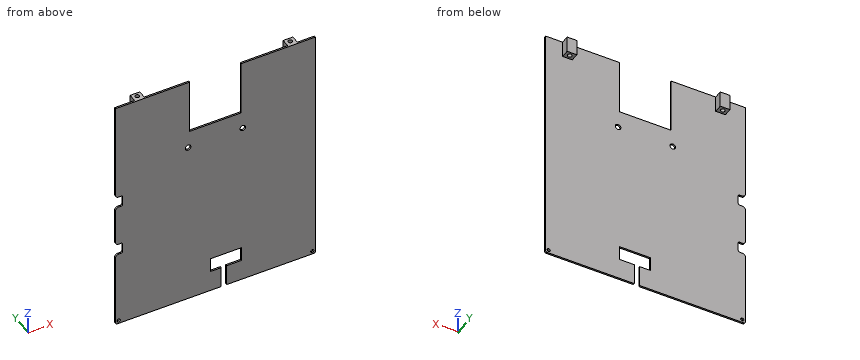
Autodesk Inventor part; units mm, degrees
ref_plane "YZ Plane" through (0, 0, 0) normal (1, 0, 0) x (0, 1, 0)
ref_plane "XZ Plane" through (0, 0, 0) normal (0, 1, 0) x (-1, 0, 0)
ref_plane "XY Plane" through (0, 0, 0) normal (0, 0, 1) x (1, 0, 0)
sketch "Sketch1" plane through (0, 0, 0) normal (0, 1, 0) x (-1, 0, 0)
  line L0 (-90.1493, 193.0734) -> (34.8507, 193.0734) construction
  line L1 (34.8507, 193.0734) -> (34.8507, 51.5734) construction
  line L2 (34.8507, 51.5734) -> (28.8507, 51.5734) construction
  line L3 (28.8507, 51.5734) -> (28.8507, 31.5734) construction
  line L4 (34.8507, 31.5734) -> (28.8507, 31.5734) construction
  line L5 (34.8507, 31.5734) -> (34.8507, -109.9266) construction
  line L6 (34.8507, -109.9266) -> (-90.1493, -109.9266) construction
  line L7 (-90.1493, -109.9266) -> (-90.1493, 31.5734) construction
  line L8 (-90.1493, 31.5734) -> (-84.1493, 31.5734) construction
  line L9 (-84.1493, 51.5734) -> (-84.1493, 31.5734) construction
  line L10 (-90.1493, 51.5734) -> (-84.1493, 51.5734) construction
  line L11 (-90.1493, 51.5734) -> (-90.1493, 193.0734) construction
  line L12 (-91.6493, 194.5734) -> (-91.6493, -111.4266) construction
  line L13 (-91.6493, -111.4266) -> (36.3507, -111.4266) construction
  line L14 (36.3507, -111.4266) -> (36.3507, 194.5734) construction
  line L15 (36.3507, 194.5734) -> (-91.6493, 194.5734) construction
  circle A0 centre (-88.1493, -107.9266) radius 1.1 construction
  line L16 (-86.1493, -109.9266) -> (-90.1493, -109.9266) construction
  line L17 (-86.1493, -109.9266) -> (-86.1493, -105.9266) construction
  line L18 (-86.1493, -105.9266) -> (-90.1493, -105.9266) construction
  line L19 (-90.1493, -109.9266) -> (-90.1493, -105.9266) construction
  line L20 (34.8507, -109.9266) -> (30.8507, -109.9266) construction
  line L21 (34.8507, -105.9687) -> (34.8507, -109.9266) construction
  line L22 (34.8507, -105.9687) -> (30.8507, -105.9687) construction
  line L23 (30.8507, -105.9687) -> (30.8507, -109.9266) construction
  circle A1 centre (32.8507, -107.9687) radius 1.1 construction
  circle A2 centre (-88.1493, 191.0734) radius 1.1 construction
  line L24 (-90.1493, 189.0734) -> (-90.1493, 193.0734) construction
  line L25 (-90.1493, 189.0734) -> (-86.1493, 189.0734) construction
  line L26 (-86.1493, 189.0734) -> (-86.1493, 193.0734) construction
  line L27 (-90.1493, 193.0734) -> (-86.1493, 193.0734) construction
  circle A3 centre (32.8507, 191.0734) radius 1.1 construction
  line L28 (30.8507, 193.0734) -> (34.8507, 193.0734) construction
  line L29 (30.8507, 193.0734) -> (30.8507, 189.0734) construction
  line L30 (30.8507, 189.0734) -> (34.8507, 189.0734) construction
  line L31 (34.8507, 193.0734) -> (34.8507, 189.0734) construction
  point P0 (0, 0)
  point P1 (0, 0)
sketch "Sketch2" plane through (0, 0, 0) normal (0, 1, 0) x (-1, 0, 0)
  line L0 (-89.7618, 28.8226) -> (-89.7618, 191.8096)
  line L1 (-88.7618, 192.8096) -> (33.3754, 192.8096)
  line L2 (34.3754, 191.8096) -> (34.3754, -108.6932)
  line L3 (-89.7618, -108.6932) -> (-89.7618, 28.8226)
  circle A0 centre (-87.7618, -107.6932) radius 1
  circle A1 centre (32.3754, -107.6932) radius 1
  line L4 (34.3754, 28.9308) -> (34.3754, -108.6932)
  circle A2 centre (-87.7618, 190.8096) radius 1
  circle A3 centre (32.3754, 190.8096) radius 1
  arc A4 (34.3754, 191.8096) -> (33.3754, 192.8096) centre (33.3754, 191.8096) ccw
  arc A5 (-88.7618, 192.8096) -> (-89.7618, 191.8096) centre (-88.7618, 191.8096) ccw
  arc A6 (-89.7618, -108.6932) -> (-88.7618, -109.6932) centre (-88.7618, -108.6932) ccw
  arc A7 (33.3754, -109.6932) -> (34.3754, -108.6932) centre (33.3754, -108.6932) ccw
  line L5 (-43.6932, 76.0582) -> (-11.6932, 76.0582)
  line L6 (-11.6932, 76.0582) -> (-11.6932, 7.0582)
  line L7 (-11.6932, 7.0582) -> (-43.6932, 7.0582)
  line L8 (-43.6932, 7.0582) -> (-43.6932, 76.0582)
  circle A8 centre (-44.6932, 80.8582) radius 1.75
  circle A9 centre (-10.6932, 80.8582) radius 1.75
  circle A10 centre (-10.6932, -3.9418) radius 1.75
  circle A11 centre (-44.6932, -3.9418) radius 1.75
  line L9 (-43.8518, -87.5066) -> (-24.58, -87.5066)
  line L10 (-24.58, -87.5066) -> (-24.58, -96.4362)
  line L11 (-43.8518, -96.4362) -> (-43.8518, -87.5066)
  line L12 (-34.6195, -96.4362) -> (-34.6195, -109.6932)
  line L13 (-31.2888, -109.6932) -> (-31.2888, -96.4362)
  line L14 (-24.58, -96.4362) -> (-31.2888, -96.4362)
  line L15 (-34.6195, -96.4362) -> (-43.8518, -96.4362)
  line L16 (33.3754, -109.6932) -> (-31.2888, -109.6932)
  line L17 (-34.6195, -109.6932) -> (-88.7618, -109.6932)
  line L18 (34.0825, -109.4003) -> (-89.4689, 192.5167) construction
  line L19 (-89.4689, -109.4003) -> (34.0825, 192.5167) construction
  line L20 (-27.6932, 41.5582) -> (9.3943, 41.5582) construction
  point P0 (0, 0)
  point P1 (-89.7618, 188.8096)
  point P2 (-85.7618, 192.8096)
  point P3 (-89.7618, 192.8096)
  dimension "d3" = 1
  dimension "d47" = 69
  dimension "d48" = 32
  dimension "d52" = 34.5
  dimension "d53" = 16
  dimension "d54" = 3.5
  dimension "d55" = 3.5
  dimension "d56" = 3.5
  dimension "d57" = 3.5
  dimension "d59" = 0
  dimension "d62" = 0
  dimension "d64" = 0
  dimension "d65" = 0
  dimension "d66" = 11
  dimension "d67" = 4.8
  dimension "d68" = 1
  dimension "d69" = 1
  dimension "d87" = 2
  dimension "d88" = 2
  dimension "d89" = 2
  dimension "d90" = 2
  dimension "d91" = 2
  dimension "d92" = 2
  dimension "d93" = 2
  dimension "d94" = 2
  dimension "d95" = 2
  dimension "d96" = 2
  dimension "d97" = 2
  dimension "d98" = 2
extrude "Extrusion1" add sketch "Sketch2" along normal blind 1
ref_plane "Work Plane1" through (-33.3754, 0, 41.5582) normal (0, 0, 1) x (1, 0, 0)
sketch "Sketch4" plane through (0, 1, 0) normal (0, 1, 0) x (1, 0, 0)
  line L0 (79.1186, -31.5582) -> (73.1186, -31.5582)
  line L1 (73.1186, -31.5582) -> (73.1186, -51.5582)
  line L2 (73.1186, -51.5582) -> (79.1186, -51.5582)
  line L3 (79.1186, -51.5582) -> (79.1186, -31.5582)
  line L4 (117.2493, -41.5582) -> (-61.9507, -41.5582)
  line L5 (-15.9231, -31.5582) -> (-21.9231, -31.5582)
  line L6 (-21.9231, -31.5582) -> (-21.9231, -51.5582)
  line L7 (-21.9231, -51.5582) -> (-15.9231, -51.5582)
  line L8 (-15.9231, -51.5582) -> (-15.9231, -31.5582)
  dimension "d10" = 6
  dimension "d11" = 20
  dimension "d12" = 10
  dimension "d13" = 6
  dimension "d14" = 20
  dimension "d15" = 10
extrude "Extrusion2" add sketch "Sketch4" along normal blind 5
sketch "Sketch6" plane through (-21.9231, 1, 51.5582) normal (0, 0, 1) x (1, 0, 0)
  line L0 (0, 5) -> (6, 5)
  line L1 (0, 0) -> (0, 5)
  line L2 (95.0417, 5) -> (101.0417, 5)
  line L3 (95.0417, 0) -> (95.0417, 5)
  point P0 (21.9231, -1)
  point P1 (3, 2.5)
  point P2 (98.0417, 2.5)
  dimension "d22" = 2.5
  dimension "d23" = 3
  dimension "d24" = 2.5
  dimension "d25" = 3
hole "Hole1" at (-18.9231, 3.5, 51.5582) at (76.1186, 3.5, 51.5582) direction (0, 0, -1) diameter 2.6 depth 5 countersink diameter 5 countersink angle 82
sketch "Sketch7" plane through (-18.9231, 3.5, 46.5582) normal (0, 0, 1) x (1, 0, 0)
  circle A0 centre (0, 0) radius 1.3
  point P0 (18.9231, -3.5)
hole "Hole2" at (-18.9231, 3.5, 46.5582) direction (0, 0, -1) diameter 2.6 depth 15 tip angle 118
sketch "Sketch8" plane through (76.1186, 3.5, 46.5582) normal (0, 0, 1) x (1, 0, 0)
  circle A0 centre (0, 0) radius 1.3
  point P0 (-76.1186, -3.5)
hole "Hole3" at (76.1186, 3.5, 46.5582) direction (0, 0, -1) diameter 2.6 depth 15 tip angle 118
sketch "Sketch9" plane through (0, 0, 0) normal (0, -1, 0) x (1, 0, 0)
  line L0 (-34.3754, -108.6932) -> (-34.3754, 191.8096)
  line L1 (-34.3754, 137.8096) -> (-30.8754, 137.8096)
  line L2 (-29.8754, 136.8096) -> (-29.8754, 131.8096)
  line L3 (-30.8754, 130.8096) -> (-34.3754, 130.8096)
  line L4 (-34.3754, 130.8096) -> (-34.3754, 137.8096)
  line L5 (-34.3754, 104.8096) -> (-30.8754, 104.8096)
  line L6 (-29.8754, 103.8096) -> (-29.8754, 98.8096)
  line L7 (-30.8754, 97.8096) -> (-34.3754, 97.8096)
  line L8 (-34.3754, 97.8096) -> (-34.3754, 104.8096)
  line L9 (-34.3754, -21.1904) -> (-30.8754, -21.1904)
  line L10 (-29.8754, -22.1904) -> (-29.8754, -27.1904)
  line L11 (-30.8754, -28.1904) -> (-34.3754, -28.1904)
  line L12 (-34.3754, -28.1904) -> (-34.3754, -21.1904)
  line L13 (-34.3754, -54.1904) -> (-30.8754, -54.1904)
  line L14 (-29.8754, -55.1904) -> (-29.8754, -60.1904)
  line L15 (-30.8754, -61.1904) -> (-34.3754, -61.1904)
  line L16 (-34.3754, -61.1904) -> (-34.3754, -54.1904)
  line L17 (-33.3754, 192.8096) -> (88.7618, 192.8096)
  arc A0 (-29.8754, 136.8096) -> (-30.8754, 137.8096) centre (-30.8754, 136.8096) ccw
  arc A1 (-30.8754, 130.8096) -> (-29.8754, 131.8096) centre (-30.8754, 131.8096) ccw
  arc A2 (-29.8754, 103.8096) -> (-30.8754, 104.8096) centre (-30.8754, 103.8096) ccw
  arc A3 (-30.8754, 97.8096) -> (-29.8754, 98.8096) centre (-30.8754, 98.8096) ccw
  arc A4 (-29.8754, -22.1904) -> (-30.8754, -21.1904) centre (-30.8754, -22.1904) ccw
  arc A5 (-30.8754, -28.1904) -> (-29.8754, -27.1904) centre (-30.8754, -27.1904) ccw
  arc A6 (-29.8754, -55.1904) -> (-30.8754, -54.1904) centre (-30.8754, -55.1904) ccw
  arc A7 (-30.8754, -61.1904) -> (-29.8754, -60.1904) centre (-30.8754, -60.1904) ccw
  point P0 (0, 0)
  point P1 (-29.8754, 97.8096)
  point P2 (-29.8754, 104.8096)
  point P3 (-29.8754, -28.1904)
  point P4 (-29.8754, -21.1904)
  point P5 (-29.8754, -61.1904)
  point P6 (-29.8754, -54.1904)
  dimension "d70" = 55
  dimension "d71" = 7
  dimension "d72" = 7
  dimension "d73" = 26
  dimension "d74" = 26
  dimension "d75" = 7
  dimension "d76" = 7
  dimension "d77" = 119
  dimension "d78" = 4.5
  dimension "d79" = 4.5
  dimension "d80" = 1
  dimension "d81" = 1
extrude "Extrusion3" cut sketch "Sketch9" against normal through all
fillet "Fillet1" radius 2 8 edges at (-34.3754, 0.5, 137.8096) (-34.3754, 0.5, 130.8096) (-34.3754, 0.5, 104.8096) (-34.3754, 0.5, 97.8096) (-34.3754, 0.5, -21.1904) (-34.3754, 0.5, -28.1904) (-34.3754, 0.5, -54.1904) (-34.3754, 0.5, -61.1904)
sketch "Sketch11" plane through (0, 0, 0) normal (0, -1, 0) x (1, 0, 0)
  line L0 (-34.3754, 139.8096) -> (-34.3754, 191.8096)
  line L1 (-34.3754, 178.177) -> (-25.2482, 178.177)
  line L2 (-25.2482, 178.177) -> (-25.2482, 158.3724)
  line L3 (-25.2482, 158.3724) -> (-34.3754, 158.3724)
  line L4 (-34.3754, 158.3724) -> (-34.3754, 178.177)
  point P0 (0, 0)
extrude "Extrusion5" cut sketch "Sketch11" against normal through all
fillet "Fillet2" radius 3 4 edges at (-34.3754, 0.5, 178.177) (-25.2482, 0.5, 178.177) (-25.2482, 0.5, 158.3724) (-34.3754, 0.5, 158.3724)
sketch "Sketch10" plane through (-33.3754, 0, 41.5582) normal (0, 0, 1) x (1, 0, 0)
  line L0 (158.018, -104.466) -> (-19.6119, -104.466)
  line L1 (-19.6119, -104.466) -> (-19.6119, 75.8038)
  line L2 (-19.6119, 75.8038) -> (158.018, 75.8038)
  line L3 (158.018, 75.8038) -> (158.018, -104.466)
  point P0 (33.3754, 0)
extrude "Extrusion4" cut sketch "Sketch10" along normal through all
properties part number "Screen Plate"
Model file for the job. Use its own axes, mm. Coordinates: 2 decimals unless noted, no trailing zeros. Write each loop counter-clockwise with the first axis right and the second up, starting at its lowest first coordinate (ties: lowest second). Pieces come first, ordered by that corner, then holes. Notation, with made-up numbers: (-28, 89.5) - (-8, 89.5) arc R36 cw to (-8, 128.5) - close; hole circle Ø10 at (-5, 71). An arc over 180 degrees is marked (long way). One line per item, written item: value. Start each with the question number.
1. Slice it at A-A (y = 3.5). Write the cut outline in (x, z).
2. Flat gauge pins, fed straight in: pin 1 (12 mm diameter, centred on x = 33, z = -65, fed in from -Y); pin 2 (1.1 mm diameter, centred on x = 41, y = 0.5, fed in from +Z); pin 3 (0.8 mm diameter, centred on y = 0.5, z = -56.5, fed in from -X); pin 4 (4 mm diameter, centred on x = 44.69, z = -3.94, fed in from +Y). Where does each tip first touch, or does it go through?
3. Slice it at C-C (z = 0.5). Write the cut outline in (x, y).
4. Probe line 1 (X direction, y = 3.5, z = 37.75); line 2 (Y direction, x = 82, z = 2.5); line 3 (Z direction, x = -21.5, y = 4.6). List the from-to ranges inside material, lowest first. Write a range as from..to.
5. Slice it at B-B (z = 19). Write the cut outline in (x, y).
6. Slice it at D-D (x = 4). Write the cut outline in (y, z), plus the area to 3 significant figures.
Answers below:
1. outline: (-21.92, 31.56) - (-20.22, 31.56) - (-20.22, 41.56) - (-21.92, 41.56) - close; (-17.62, 31.56) - (-15.92, 31.56) - (-15.92, 41.56) - (-17.62, 41.56) - close; (73.12, 31.56) - (74.82, 31.56) - (74.82, 41.56) - (73.12, 41.56) - close; (77.42, 31.56) - (79.12, 31.56) - (79.12, 41.56) - (77.42, 41.56) - close
2. pin 1: stops at y = 0
2. pin 2: stops at z = 7.06
2. pin 3: stops at x = -29.88
2. pin 4: stops at y = 1
3. outline: (-34.38, 0) - (89.76, 0) - (89.76, 1) - (-34.38, 1) - close
4. line 1: x = -21.92..-20.22, -17.62..-15.92, 73.12..74.82, 77.42..79.12
4. line 2: y = 0..1
4. line 3: z = 31.56..41.56
5. outline: (-34.38, 0) - (11.69, 0) - (11.69, 1) - (-34.38, 1) - close; (43.69, 0) - (89.76, 0) - (89.76, 1) - (43.69, 1) - close
6. outline: (0, -109.69) - (1, -109.69) - (1, 41.56) - (0, 41.56) - close
6. area: 151 mm^2
